Can you work these out from the model? Positions are in its coordinate system, mm. Coordinates: 2 decimals unless noted, no trailing zeros. Loops run counter-clockwise (first coordinate to the right, second up) from the corner with the lowest first, then second, coordinate; pieces in that order, holes last. Notation, with made-up numbers: (-5.75, 52.25) -> (22.25, 52.25) arc R24 ccw to (22.25, 73.25) -> close; hole circle Ø4 at (20.25, -28). An arc over 180 degrees is marked (long way). Put each result on its own line as item: value. Start each with the question number.
Item 1: If we section it at B-B on y = 19: Please give me the cut outline in (x, z), plus the area to 3 significant figures.
Item 2: If we section it at D-D on z = 0.6: State how many separate pieces and enclosed holes the cut face has, plus the area to 3 significant figures.
Item 3: If we section it at C-C on x = 6.5: Please give me the cut outline in (y, z).
Item 4: Please list where these lines run through material, in increasing order: L1, parallel to Y at x = -15.5, z = 0.55; L2, parallel to X at y = -41, z = 0.1; L3, parallel to X at y = 9, z = 1.25. Write a range as from..to.
Item 5: If we section it at A-A on y = -51: Please give me the cut outline in (x, z).
Item 6: Will these pins go through, and if not, where does the flat tip stop? P1, Ø1, axis at y = 3.5, z = 0.5, coming from the -X side; P2, Ø1.1, axis at x = 40, z = 0.5, coming from the -Y side.
Autodesk Inventor part; units mm, degrees
ref_plane "YZ Plane" through (0, 0, 0) normal (1, 0, 0) x (0, 1, 0)
ref_plane "XZ Plane" through (0, 0, 0) normal (0, 1, 0) x (-1, 0, 0)
ref_plane "XY Plane" through (0, 0, 0) normal (0, 0, 1) x (1, 0, 0)
sketch "スケッチ1" plane through (0, 0, 0) normal (0, 0, 1) x (1, 0, 0)
  circle A0 centre (0, 0) radius 11
  line L0 (-0.3073, 13.5) -> (26.6927, 13.5) construction
  line L1 (26.6927, 13.5) -> (26.6927, -13.5) construction
  line L2 (26.6927, -13.5) -> (-0.3073, -13.5) construction
  line L3 (-0.3073, -13.5) -> (-0.3073, 13.5) construction
  line L4 (-0.3073, 13.5) -> (26.6927, -13.5) construction
  line L5 (26.6927, 13.5) -> (-0.3073, -13.5) construction
  line L6 (-12, 16) -> (39.5, 16) construction
  line L7 (39.5, 16) -> (39.5, -16) construction
  line L8 (39.5, -16) -> (-12, -16) construction
  line L9 (-12, -16) -> (-12, 16) construction
  line L10 (-12, 16) -> (39.5, -16) construction
  line L11 (39.5, 16) -> (-12, -16) construction
  circle A1 centre (-0.3073, 13.5) radius 1.35
  arc A2 (0, 16) -> (-12, 10.583) centre (0, 0) ccw construction
  line L12 (-12, 0) -> (39.5, 0)
  circle A3 centre (26.6927, 13.5) radius 1.35
  arc A4 (-12, -10.583) -> (0, -16) centre (0, 0) ccw construction
  circle A5 centre (-0.3073, -13.5) radius 1.35
  circle A6 centre (26.6927, -13.5) radius 1.35
  arc A7 (0, 16.05) -> (-12.05, 10.6019) centre (0, 0) ccw
  line L13 (0, 16.05) -> (39.55, 16.05)
  line L14 (39.55, 16.05) -> (39.55, 13.3)
  line L15 (-12.05, 10.6019) -> (-12.05, 0)
  arc A8 (-11.5146, 11.1811) -> (-12.05, 9.86) centre (-11.0677, 10.2309) ccw
  line L16 (-12.05, 10.6019) -> (-11.0677, 10.2309) construction
  arc A9 (39.55, 14.5651) -> (38.0651, 16.05) centre (38.8075, 15.3075) ccw
  line L17 (38.8075, 15.3075) -> (39.55, 16.05) construction
  arc A10 (-12.05, -10.6019) -> (0, -16.05) centre (0, 0) ccw
  line L18 (0, -16.05) -> (39.55, -16.05)
  line L19 (-12.05, -10.6019) -> (-12.05, 0)
  arc A11 (-12.05, -9.86) -> (-11.5146, -11.1811) centre (-11.0677, -10.2309) ccw
  arc A12 (38.0651, -16.05) -> (39.55, -14.5651) centre (38.8075, -15.3075) ccw
  line L20 (39.55, 13.3) -> (42.05, 13.3)
  line L21 (42.05, 13.3) -> (42.05, -1.8)
  line L22 (42.05, -1.8) -> (39.55, -1.8)
  line L23 (39.55, -1.8) -> (39.55, -14.5651)
  line L24 (39.5, 13.25) -> (42, 13.25) construction
  line L25 (42, 13.25) -> (42, -1.75) construction
  line L26 (42, -1.75) -> (39.5, -1.75) construction
  line L27 (42, 5.75) -> (39.5, 5.75) construction
  arc A13 (42.05, 11.8151) -> (40.5651, 13.3) centre (41.3075, 12.5575) ccw
  line L28 (41.3075, 12.5575) -> (42.05, 13.3) construction
  arc A14 (40.5651, -1.8) -> (42.05, -0.3151) centre (41.3075, -1.0575) ccw
  circle A15 centre (-15.5, 19) radius 1.6
  line L29 (-18, 22) -> (-13, 22) construction
  line L30 (-13, 22) -> (-13, -10.5) construction
  line L31 (-13, -10.5) -> (-18, -10.5) construction
  line L32 (-18, -10.5) -> (-18, 22) construction
  line L33 (-18, 22) -> (-13, -10.5) construction
  line L34 (-13, 22) -> (-18, -10.5) construction
  line L35 (-18, 5.75) -> (-13, 5.75) construction
  line L36 (-15.5, 22) -> (-15.5, -10.5) construction
  line L37 (-18, 13.25) -> (-15.5, 13.25) construction
  line L38 (-15.5, 13.25) -> (-15.5, -1.75) construction
  line L39 (-15.5, -1.75) -> (-18, -1.75) construction
  line L40 (-18, 13.25) -> (-15.5, -1.75) construction
  line L41 (-15.5, 13.25) -> (-18, -1.75) construction
  line L42 (-15.45, -1.8) -> (-18.05, -1.8)
  line L43 (-18.05, -1.8) -> (-18.05, 13.3)
  line L44 (-18.05, 13.3) -> (-15.45, 13.3)
  line L45 (-15.45, 13.3) -> (-15.45, -1.8)
  line L46 (-15.45, -1.8) -> (-18.05, 13.3) construction
  line L47 (-18.05, -1.8) -> (-15.45, 13.3) construction
  line L48 (-16.75, 13.3) -> (-16.75, -1.8) construction
  arc A16 (-18.05, 13.3) -> (-18.05, 11.2) centre (-18.05, 12.25) ccw
  arc A17 (-15.45, 11.2) -> (-15.45, 13.3) centre (-15.45, 12.25) ccw
  arc A18 (-18.05, 0.3) -> (-18.05, -1.8) centre (-18.05, -0.75) ccw
  arc A19 (-15.45, -1.8) -> (-15.45, 0.3) centre (-15.45, -0.75) ccw
  circle A20 centre (-15.5, -7.5) radius 1.6
  line L49 (13.1927, 16) -> (13.1927, -16) construction
  circle A21 centre (42, 19) radius 1.6
  line L50 (39.5, 22) -> (44.5, 22) construction
  line L51 (44.5, 22) -> (44.5, -10.5) construction
  line L52 (44.5, -10.5) -> (39.5, -10.5) construction
  line L53 (39.5, 22) -> (44.5, -10.5) construction
  line L54 (44.5, 22) -> (39.5, -10.5) construction
  line L55 (42, 22) -> (42, -10.5) construction
  circle A22 centre (42, -7.5) radius 1.6
  line L56 (-12, 23.25) -> (-12, 18.25) construction
  line L57 (-18, 24.5) -> (44.5, 24.5)
  line L58 (-18, 24.5) -> (-23, 22)
  line L59 (44.5, 24.5) -> (47.5, 22)
  line L60 (-23, 22) -> (-23, -10.75)
  line L61 (47.5, 22) -> (47.5, -18.25)
  line L62 (47.5, -18.25) -> (76.5, -33.25)
  line L63 (-23, -10.75) -> (-33.5, -16)
  line L64 (-33.5, -16) -> (-33.5, -96.5)
  line L65 (76.5, -33.25) -> (76.5, -93.8101)
  line L66 (76.5, -93.8101) -> (23, -104.5)
  line L67 (23, -104.5) -> (-17, -104.5)
  line L68 (-17, -104.5) -> (-33.5, -96.5)
  circle A23 centre (-12, -99.5) radius 1.6
  circle A24 centre (3, -99.5) radius 1.6
  line L69 (-17, -104.5) -> (-17, -94.5) construction
  line L70 (-17, -94.5) -> (23, -94.5) construction
  line L71 (23, -94.5) -> (23, -104.5) construction
  line L72 (-17, -99.5) -> (23, -99.5) construction
  line L73 (3, -94.5) -> (3, -104.5) construction
  circle A25 centre (18, -99.5) radius 1.6
  circle A26 centre (-13.5, -61.75) radius 1.6
  line L74 (-23.5, -65.75) -> (66.5, -65.75)
  line L75 (66.5, -65.75) -> (66.5, -84.5)
  line L76 (66.5, -84.5) -> (-23.5, -84.5)
  line L77 (-23.5, -84.5) -> (-23.5, -65.75)
  line L78 (-23.5, -33.25) -> (66.5, -33.25)
  line L79 (66.5, -33.25) -> (66.5, -57.75)
  line L80 (66.5, -57.75) -> (-23.5, -57.75)
  line L81 (-23.5, -57.75) -> (-23.5, -33.25)
  circle A27 centre (-13.5, -61.75) radius 4 construction
  line L82 (-9.8584, -97.6093) -> (-9.2918, -98.5907)
  line L83 (-9.2918, -100.4093) -> (-9.8584, -101.3907)
  line L84 (-11.4334, -102.3) -> (-12.5666, -102.3)
  line L85 (-14.1416, -101.3907) -> (-14.7082, -100.4093)
  line L86 (-14.7082, -98.5907) -> (-14.1416, -97.6093)
  line L87 (-12.5666, -96.7) -> (-11.4334, -96.7)
  arc A28 (-9.8584, -97.6093) -> (-11.4334, -96.7) centre (-10.9084, -97.6093) ccw
  arc A29 (-12.5666, -96.7) -> (-14.1416, -97.6093) centre (-13.0916, -97.6093) ccw
  arc A30 (-14.7082, -98.5907) -> (-14.7082, -100.4093) centre (-14.1832, -99.5) ccw
  arc A31 (-14.1416, -101.3907) -> (-12.5666, -102.3) centre (-13.0916, -101.3907) ccw
  arc A32 (-11.4334, -102.3) -> (-9.8584, -101.3907) centre (-10.9084, -101.3907) ccw
  arc A33 (-9.2918, -100.4093) -> (-9.2918, -98.5907) centre (-9.8168, -99.5) ccw
  arc A34 (5.7082, -100.4093) -> (5.7082, -98.5907) centre (5.1832, -99.5) ccw
  line L88 (5.1416, -97.6093) -> (5.7082, -98.5907)
  line L89 (5.7082, -100.4093) -> (5.1416, -101.3907)
  arc A35 (3.5666, -102.3) -> (5.1416, -101.3907) centre (4.0916, -101.3907) ccw
  arc A36 (5.1416, -97.6093) -> (3.5666, -96.7) centre (4.0916, -97.6093) ccw
  line L90 (2.4334, -96.7) -> (3.5666, -96.7)
  arc A37 (2.4334, -96.7) -> (0.8584, -97.6093) centre (1.9084, -97.6093) ccw
  line L91 (0.2918, -98.5907) -> (0.8584, -97.6093)
  arc A38 (0.2918, -98.5907) -> (0.2918, -100.4093) centre (0.8168, -99.5) ccw
  line L92 (0.8584, -101.3907) -> (0.2918, -100.4093)
  arc A39 (0.8584, -101.3907) -> (2.4334, -102.3) centre (1.9084, -101.3907) ccw
  line L93 (3.5666, -102.3) -> (2.4334, -102.3)
  arc A40 (20.7082, -100.4093) -> (20.7082, -98.5907) centre (20.1832, -99.5) ccw
  line L94 (20.1416, -97.6093) -> (20.7082, -98.5907)
  line L95 (20.7082, -100.4093) -> (20.1416, -101.3907)
  arc A41 (18.5666, -102.3) -> (20.1416, -101.3907) centre (19.0916, -101.3907) ccw
  arc A42 (20.1416, -97.6093) -> (18.5666, -96.7) centre (19.0916, -97.6093) ccw
  line L96 (17.4334, -96.7) -> (18.5666, -96.7)
  arc A43 (17.4334, -96.7) -> (15.8584, -97.6093) centre (16.9084, -97.6093) ccw
  line L97 (15.2918, -98.5907) -> (15.8584, -97.6093)
  arc A44 (15.2918, -98.5907) -> (15.2918, -100.4093) centre (15.8168, -99.5) ccw
  line L98 (15.8584, -101.3907) -> (15.2918, -100.4093)
  arc A45 (15.8584, -101.3907) -> (17.4334, -102.3) centre (16.9084, -101.3907) ccw
  line L99 (18.5666, -102.3) -> (17.4334, -102.3)
  point P0 (13.1927, 0)
  point P1 (-15.5, 5.75)
  point P2 (-16.75, 5.75)
  point P3 (13.1927, 0)
  point P4 (42, 5.75)
  point P5 (42, 5.75)
  point P6 (-18.05, 0.3)
  point P7 (-15.45, 0.3)
  point P8 (42.05, -0.3151)
  point P9 (40.5651, -1.8)
  point P10 (-10.3834, -96.7)
  point P11 (-13.6166, -96.7)
  point P12 (-15.2332, -99.5)
  point P13 (-13.6166, -102.3)
  point P14 (-10.3834, -102.3)
  point P15 (-8.7668, -99.5)
  point P16 (-13.6166, -96.7)
  point P17 (-15.2332, -99.5)
  point P18 (-8.7668, -99.5)
  point P19 (3, -99.5)
  point P20 (6.2332, -99.5)
  point P21 (6.2332, -99.5)
  point P22 (4.6166, -96.7)
  point P23 (4.6166, -102.3)
  point P24 (3, -99.5)
  point P25 (3, -99.5)
  point P26 (1.3834, -96.7)
  point P27 (1.3834, -96.7)
  point P28 (-0.2332, -99.5)
  point P29 (-0.2332, -99.5)
  point P30 (1.3834, -102.3)
  point P31 (18, -99.5)
  point P32 (21.2332, -99.5)
  point P33 (21.2332, -99.5)
  point P34 (19.6166, -96.7)
  point P35 (19.6166, -102.3)
  point P36 (18, -99.5)
  point P37 (18, -99.5)
  point P38 (16.3834, -96.7)
  point P39 (16.3834, -96.7)
  point P40 (14.7668, -99.5)
  point P41 (14.7668, -99.5)
  point P42 (16.3834, -102.3)
  dimension "d0" = 22
  dimension "d1" = 27
  dimension "d2" = 27
  dimension "d5" = 32
  dimension "d8" = 2.7
  dimension "d9" = 16
  dimension "d10" = 2.7
  dimension "d13" = 12
  dimension "d16" = 0.05
  dimension "d17" = 1.05
  dimension "d18" = 0.05
  dimension "d19" = 1.05
  dimension "d21" = 15
  dimension "d23" = 0.05
  dimension "d24" = 0.05
  dimension "d25" = 0.05
  dimension "d26" = 1.05
  dimension "d27" = 3.2
  dimension "d28" = 5
  dimension "d29" = 2.5
  dimension "d30" = 15
  dimension "d32" = 2.6
  dimension "d33" = 15.1
  dimension "d34" = 1.05
  dimension "d35" = 26.5
  dimension "d36" = 5.5
  dimension "d37" = 2.5
  dimension "d38" = 3.2
  dimension "d39" = 5
  dimension "d40" = 32.5
  dimension "d41" = 26.5
  dimension "d55" = 5
  dimension "d56" = 3
  dimension "d57" = 20.5
  dimension "d60" = 40
  dimension "d61" = 8
  dimension "d63" = 3.2
  dimension "d64" = 3.2
  dimension "d66" = 10
  dimension "d70" = 30
  dimension "d71" = 3.2
  dimension "d72" = 32.75
  dimension "d73" = 20
  dimension "d74" = 8
  dimension "d75" = 10
  dimension "d77" = 10
  dimension "d78" = 10
  dimension "d87" = 1.05
  dimension "d88" = 360
  dimension "d89" = 5.6
  dimension "d92" = 15
  dimension "d97" = 120.5
  dimension "d98" = 1
  dimension "d100" = 110
  dimension "d101" = 2.5
extrude "押し出し1" add sketch "スケッチ1" along normal blind 2 contours L57 L59 L61 L62 L65 L66 L67 L68 L64 L63 L60 L58 | L82 A33 L83 A32 L84 A31 L85 A30 L86 A29 L87 A28 | L89 A35 L93 A39 L92 A38 L91 A37 L90 A36 L88 A34 | L95 A41 L99 A45 L98 A44 L97 A43 L96 A42 L94 A40
fillet "フィレット1" radius 2 12 edges at (-17, -104.5, 1) (-33.5, -96.5, 1) (-33.5, -16, 1) (-23, -10.75, 1) (23, -104.5, 1) (76.5, -93.8101, 1) (76.5, -33.25, 1) (47.5, -18.25, 1) (47.5, 22, 1) (44.5, 24.5, 1) (-23, 22, 1) (-18, 24.5, 1)
fillet "フィレット2" radius 2 8 edges at (-23.5, -33.25, 1) (-23.5, -57.75, 1) (66.5, -57.75, 1) (66.5, -33.25, 1) (-23.5, -84.5, 1) (-23.5, -65.75, 1) (66.5, -84.5, 1) (66.5, -65.75, 1)
equation "\"d10\" = d8"
equation "\"d16\" = d15"
equation "\"d18\" = d15"
equation "\"d19\" = d17"
equation "\"d23\" = d15"
equation "\"d24\" = d23"
equation "\"d25\" = d15"
equation "\"d26\" = d17"
properties part number "Trunk_upper_flank_frame" material "GFRP"
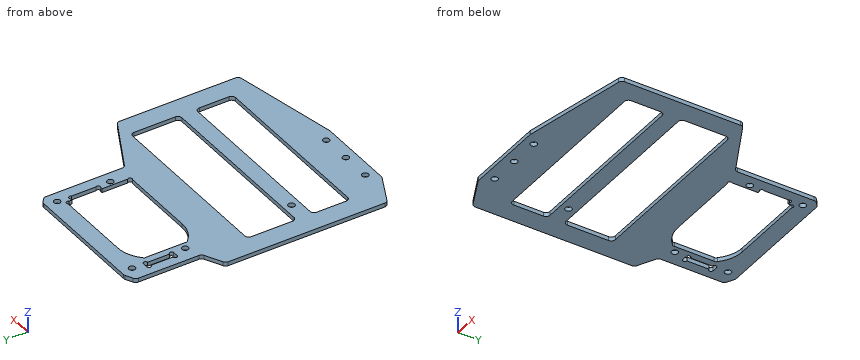
Solutions:
1. outline: (-23, 0) -> (-17.1, 0) -> (-17.1, 2) -> (-23, 2) -> close; (-13.9, 0) -> (40.4, 0) -> (40.4, 2) -> (-13.9, 2) -> close; (43.6, 0) -> (47.5, 0) -> (47.5, 2) -> (43.6, 2) -> close
1. area: 128 mm^2
2. separate pieces: 1
2. enclosed holes: 12
2. area: 6,320 mm^2
3. outline: (-104.5, 0) -> (-84.5, 0) -> (-84.5, 2) -> (-104.5, 2) -> close; (-65.75, 0) -> (-57.75, 0) -> (-57.75, 2) -> (-65.75, 2) -> close; (-33.25, 0) -> (-16.05, 0) -> (-16.05, 2) -> (-33.25, 2) -> close; (16.05, 0) -> (24.5, 0) -> (24.5, 2) -> (16.05, 2) -> close
4. L1: -104.5..-84.5, -65.75..-57.75, -33.25..-9.1, -5.9..-1.8, 13.3..17.4, 20.6..24.5
4. L2: -33.5..-23.5, 66.5..76.5
4. L3: -23..-18.05, -15.45..-12.05, 42.05..47.5
5. outline: (-33.5, 0) -> (-23.5, 0) -> (-23.5, 2) -> (-33.5, 2) -> close; (66.5, 0) -> (76.5, 0) -> (76.5, 2) -> (66.5, 2) -> close
6. P1: x = -23
6. P2: y = -101.21
